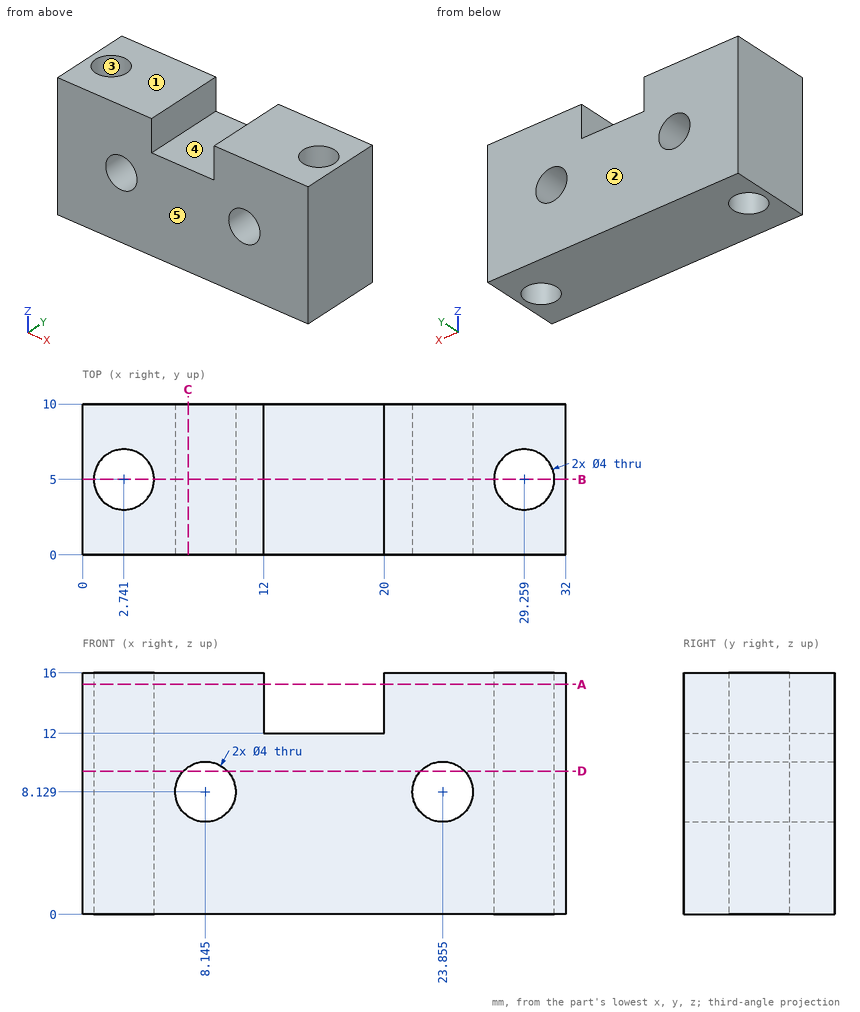
Design review of the part shown in the three views and the two pictorial views. Dimensions are in mm from the part's minimum x, y and z. A direction names the side the tool comes from. Give positions to 0.01 mm unless a question says otherwise; leave off trailing zeros. Write each loop counter-clockwise with the first axis right and the second up, starting at its lowest first coordinate (ties: lowest second). Pieces come first, ordered by that corner, then holes. Notation, with made-up numbers: M -13,72.5 L 46,72.5 A12 ccw 46,85.5 Z; hole C -20.75,-12 d7. An arc over 180 degrees is marked long. Return JSON: item names as keys, results as strings. Group by question number.
Item 1: Tool access review of the marked faces 4 and 5: name each direction out of +Z, -Z, +X, -X, +Y, -Y from which nothing blocks a thin tool from reaching the whole face with its end or side.
Item 2: Take a section at C-C (x = 7). Give the boundary of the cut face in (y, z), plus the area to 3 significant figures.
Item 3: The part is to be moulded in two halves that separate along Y. For the marked faces 1, 2 and 3, say which applies: pulls with the +Y half, pulls with the -Y half, needs draft (parallel to the pull), parting line crosses it, or undercut.
Item 4: Take a section at D-D (z = 9.5). Give the boundary of the cut face in (x, y).
Item 5: Take a section at B-B (y = 5). Give the boundary of the cut face in (x, z) (1 decimal), plus the area to 3 significant figures.
Item 6: Wall thickness on line 1 along X through (y, z) = (5.75, 11.25) (1 decimal); line 2 along X through (y, z) = (6, 5.5); line 3 along X through (y, z) = (1.5, 13.75): over which ranges is each line inside the solid? List them lowest first.
Item 7: Take a section at A-A (z = 15.25). Give the boundary of the cut face in (x, y), plus the area to 3 significant figures.
Return value:
{
 "1": {"face 4": "+Z, +Y, -Y", "face 5": "+Z, -Z, +X, -X, -Y"},
 "2": {"outline": "M 0,0 L 10,0 L 10,6.49 L 0,6.49 Z; M 0,9.77 L 10,9.77 L 10,16 L 0,16 Z", "area": "127 mm2"},
 "3": {"face 1": "needs draft", "face 2": "pulls with the +Y half", "face 3": "undercut"},
 "4": {"outline": "M 0,0 L 6.69,0 L 6.69,10 L 0,10 Z; M 9.6,0 L 22.4,0 L 22.4,10 L 9.6,10 Z; M 25.31,0 L 32,0 L 32,10 L 25.31,10 Z; hole C 2.74,5 d4; hole C 29.26,5 d4"},
 "5": {"outline": "M 0,0 L 0.7,0 L 0.7,16 L 0,16 Z; M 4.7,0 L 27.3,0 L 27.3,16 L 20,16 L 20,12 L 12,12 L 12,16 L 4.7,16 Z; M 31.3,0 L 32,0 L 32,16 L 31.3,16 Z; hole C 8.1,8.1 d4; hole C 23.9,8.1 d4", "area": "327 mm2"},
 "6": {"line 1": "x = 0 to 0.9, 4.6 to 27.4, 31.1 to 32", "line 2": "x = 0 to 1.01, 4.47 to 27.53, 30.99 to 32", "line 3": "x = 0 to 12, 20 to 32"},
 "7": {"outline": "M 0,0 L 12,0 L 12,10 L 0,10 Z; M 20,0 L 32,0 L 32,10 L 20,10 Z; hole C 2.74,5 d4; hole C 29.26,5 d4", "area": "215 mm2"}
}
